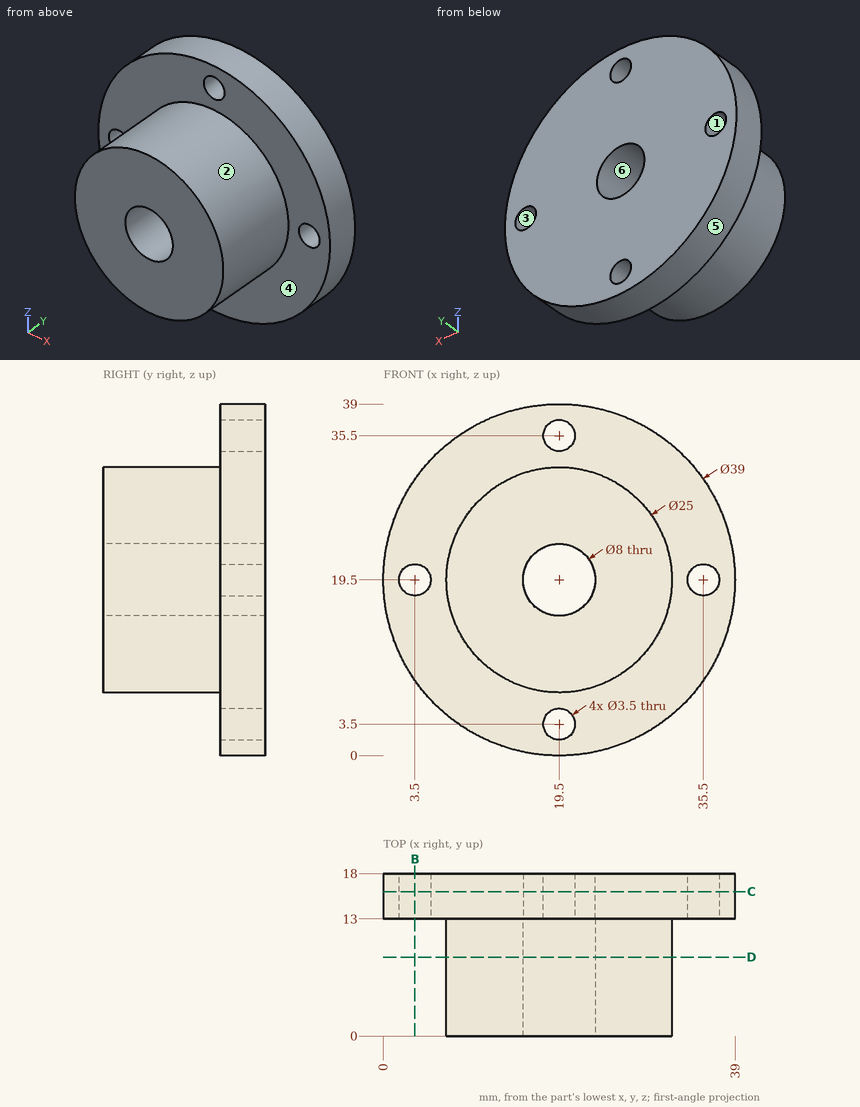
Answer from the drawing. Dimensions are ordinates in mm from the lowest x, y and z of the part. A direction names the side the tool comes from. Round coordinates to 2 decimals unless told otherwise and drop trailing zeros. Loops run counter-clockwise (first coordinate to the right, second up) from the corner with the lowest first, then second, coordinate; pieces in that order, holes last. Notation, with made-up numbers: M -6.75,87.25 L 47.25,87.25 A17 ccw 47.25,104.25 Z; hole C -0.75,13 d8. An arc over 180 degrees is marked long. One line per question, with ' | ' between items. Start each with the question number.
(1) For a pull along X with two mould halves and no side action, classify the marked faces 3, 4, 5 and 6 as released by +X, released by -X, zero draft, split by the parting line, or undercut.
(2) A cutting plane is placed at D-D on y = 8.75. Write down the section's boundary in (x, z).
(3) Find the intervals of material crossed by line 1 (Z direction, x = 19.5, y = 14.2); line 2 (Z direction, x = 19.5, y = 12.25), in increasing order.
(4) A cutting plane is placed at B-B on x = 3.5. Write down the section's boundary in (y, z).
(5) Flat-ended cylindrical pins translate along their axes: pin 1 Ø3 at (x, y) = (17.5, 3) entering from +Z; pin 2 Ø3 at (x, z) = (19.5, 35.5) entering from -Y; pin 3 Ø4 at (x, z) = (19.5, 3.5) entering from -Y; pin 4 Ø1 at (y, z) = (15.5, 26.5) entering from -X. Find the tip coordinate at first contact, or state that the pin passes through.
(6) A cutting plane is placed at C-C on y = 16. Write down the section's boundary in (x, z).
(7) A tool of negligible diameter and unlimited length cuts with its end or side. For the marked faces 1 and 2, from which of +Z, -Z, +X, -X, +Y, -Y can it reach the whole face along a straight path? Write none if from no direction.
Geometry check:
1) face 3: undercut | face 4: zero draft | face 5: split by the parting line | face 6: undercut
2) outline: C 19.5,19.5 d25; hole C 19.5,19.5 d8
3) line 1: z = 0 to 1.75, 5.25 to 15.5, 23.5 to 33.75, 37.25 to 39 | line 2: z = 7 to 15.5, 23.5 to 32
4) outline: M 13,8.35 L 18,8.35 L 18,17.75 L 13,17.75 Z; M 13,21.25 L 18,21.25 L 18,30.65 L 13,30.65 Z
5) pin 1: stops at z = 31.99 | pin 2: passes through | pin 3: stops at y = 13 | pin 4: stops at x = 1.12
6) outline: C 19.5,19.5 d39; hole C 3.5,19.5 d3.5; hole C 19.5,19.5 d8; hole C 19.5,3.5 d3.5; hole C 19.5,35.5 d3.5; hole C 35.5,19.5 d3.5
7) face 1: +Y, -Y | face 2: -Y
